from build123d import *

# Parameters (mm, degrees)
BOSS_EXTRU_1_DEPTH      = 8
ENL_V_MAT_EXTRU_1_DEPTH = 5
ESQUISSE4_W             = 5
ESQUISSE4_H             = 1
BOSS_EXTRU_3_DEPTH      = 0.48904
ESQUISSE5_W             = 1
ESQUISSE5_H             = 5
BOSS_EXTRU_4_DEPTH      = 0.48904
ESQUISSE6_W             = 1
ESQUISSE6_H             = 5
BOSS_EXTRU_5_DEPTH      = 0.48904
ESQUISSE7_W             = 1
ESQUISSE7_H             = 5
BOSS_EXTRU_6_DEPTH      = 0.48904
ESQUISSE8_W             = 5
ESQUISSE8_H             = 1
BOSS_EXTRU_7_DEPTH      = 0.48904
ESQUISSE9_W             = 5
ESQUISSE9_H             = 1
BOSS_EXTRU_8_DEPTH      = 0.48904
ESQUISSE10_W            = 3
ESQUISSE10_H            = 36.5
ENL_V_MAT_EXTRU_3_DEPTH = 99.707699801
ESQUISSE11_W            = 41.5
ESQUISSE11_H            = 3
ENL_V_MAT_EXTRU_4_DEPTH = 99.686422572
ESQUISSE12_W            = 11
ESQUISSE12_H            = 3
ENL_V_MAT_EXTRU_5_DEPTH = 99.686422572


with BuildPart() as part:
    # Esquisse1 → Boss.-Extru.1 (new body)
    with BuildSketch(Plane.XY):
        with BuildLine():
            Line((2, 0), (67, 0))
            ThreePointArc((67, 0), (68.414213562, 0.585786438), (69, 2))
            Line((69, 2), (69, 69.1))
            ThreePointArc((69, 69.1), (68.414213562, 70.514213562), (67, 71.1))
            Line((67, 71.1), (2, 71.1))
            ThreePointArc((2, 71.1), (0.585786438, 70.514213562), (0, 69.1))
            Line((0, 69.1), (0, 2))
            ThreePointArc((0, 2), (0.585786438, 0.585786438), (2, 0))
        make_face()
    extrude(amount=BOSS_EXTRU_1_DEPTH)

    # Esquisse3 → Enlèv. mat.-Extru.1 (cut)
    with BuildSketch(Plane.XY.offset(8)):
        with BuildLine():
            Line((2, 1), (67, 1))
            ThreePointArc((67, 1), (67.707106781, 1.292893219), (68, 2))
            Line((68, 2), (68, 69.1))
            ThreePointArc((68, 69.1), (67.707106781, 69.807106781), (67, 70.1))
            Line((67, 70.1), (2, 70.1))
            ThreePointArc((2, 70.1), (1.292893219, 69.807106781), (1, 69.1))
            Line((1, 69.1), (1, 2))
            ThreePointArc((1, 2), (1.292893219, 1.292893219), (2, 1))
        make_face()
    extrude(amount=-ENL_V_MAT_EXTRU_1_DEPTH, mode=Mode.SUBTRACT)

    # Esquisse4 → Boss.-Extru.3 (add)
    with BuildSketch(Plane.XZ.offset(-70.1)):
        with Locations((10.679731729, 6.5)):
            Rectangle(ESQUISSE4_W, ESQUISSE4_H)
    extrude(amount=BOSS_EXTRU_3_DEPTH)

    # Esquisse5 → Boss.-Extru.4 (add)
    with BuildSketch(Plane.ZY.offset(-68)):
        with Locations((6.5, 63.6)):
            Rectangle(ESQUISSE5_W, ESQUISSE5_H)
    extrude(amount=BOSS_EXTRU_4_DEPTH)

    # Esquisse6 → Boss.-Extru.5 (add)
    with BuildSketch(Plane(origin=(1, 0, 0), x_dir=(0, 0, -1), z_dir=(1, 0, 0))):
        with Locations((-6.5, 62.6)):
            Rectangle(ESQUISSE6_W, ESQUISSE6_H)
    extrude(amount=BOSS_EXTRU_5_DEPTH)

    # Esquisse7 → Boss.-Extru.6 (add)
    with BuildSketch(Plane(origin=(1, 0, 0), x_dir=(0, 0, -1), z_dir=(1, 0, 0))):
        with Locations((-6.5, 8.5)):
            Rectangle(ESQUISSE7_W, ESQUISSE7_H)
    extrude(amount=BOSS_EXTRU_6_DEPTH)

    # Esquisse8 → Boss.-Extru.7 (add)
    with BuildSketch(Plane(origin=(0, 1, 0), x_dir=(1, 0, 0), z_dir=(0, 1, 0))):
        with Locations((14.5, -6.5)):
            Rectangle(ESQUISSE8_W, ESQUISSE8_H)
    extrude(amount=BOSS_EXTRU_7_DEPTH)

    # Esquisse9 → Boss.-Extru.8 (add)
    with BuildSketch(Plane(origin=(0, 1, 0), x_dir=(1, 0, 0), z_dir=(0, 1, 0))):
        with Locations((47, -6.5)):
            Rectangle(ESQUISSE9_W, ESQUISSE9_H)
    extrude(amount=BOSS_EXTRU_8_DEPTH)

    # Esquisse10 → Enlèv. mat.-Extru.3 (cut, through all)
    with BuildSketch(Plane.ZY.offset(-68)):
        with Locations((6.5, 26.25)):
            Rectangle(ESQUISSE10_W, ESQUISSE10_H)
    extrude(amount=-ENL_V_MAT_EXTRU_3_DEPTH, mode=Mode.SUBTRACT)

    # Esquisse11 → Enlèv. mat.-Extru.4 (cut, through all)
    with BuildSketch(Plane.XZ.offset(-70.1)):
        with Locations((39.25, 6.5)):
            Rectangle(ESQUISSE11_W, ESQUISSE11_H)
    extrude(amount=-ENL_V_MAT_EXTRU_4_DEPTH, mode=Mode.SUBTRACT)

    # Esquisse12 → Enlèv. mat.-Extru.5 (cut, through all)
    with BuildSketch(Plane(origin=(0, 1, 0), x_dir=(1, 0, 0), z_dir=(0, 1, 0))):
        with Locations((27.5, -6.5)):
            Rectangle(ESQUISSE12_W, ESQUISSE12_H)
    extrude(amount=-ENL_V_MAT_EXTRU_5_DEPTH, mode=Mode.SUBTRACT)


solid = part.part
The model under review builds one solid part; all positions refer to its coordinate system, in mm. A direction names the side the tool comes from. Round coordinates to 2 decimals unless told otherwise and drop trailing zeros. Loops run counter-clockwise (first coordinate to the right, second up) from the corner with the lowest first, then second, coordinate; pieces in that order, holes last. Notation, with made-up numbers: (-9.5, 1.25) -> (10.5, 1.25) arc R31 ccw to (10.5, 33.25) -> close; hole circle Ø8 at (36.25, 16.25). An arc over 180 degrees is marked (long way). One line per question, with ' | ' between items. Start each with the question number.
Item 1: Add section B-B, the plane x = 61. Write out the cut boundary in (y, z).
Item 2: Machinability: for faces 4 (the face through (54.9, 0.8, 8)), 5 (the face through (34, 1, 6)), which of the approach directions +Z, -Z, +X, -X, +Y, -Y give a long, thin tool a straight path to every point of the face, cutting with its end or side? Answer none if there is none.
Item 3: Add section C-C, the plane y = 36. Write out the cut boundary in (x, z).
Item 4: Draft analysis for pull direction Y (two halves, no side actions). For faces 1 (the face through (68.4, 0.57, 3.94)), 2 (the face through (34, 36, 3)), 3 (the face through (34, 36, 0)), state which applies: +Y half, -Y half, draft (parallel to the pull), parting line (faces both ways), or undercut.
Item 5: Add section A-A, the plane z = 4. Write out the cut boundary in (x, y), then the cut area to 3 significant figures.
Item 6: For pin 1 (0.8 mm diameter, centred on x = 30, y = 70.5, fed in from +Z); pin 2 (1.5 mm diameter, centred on x = 59, y = 10.5, fed in from +Z); pin 3 (0.8 mm diameter, centred on x = 68.5, z = 6, fed in from +Y), all flat-tipped, find the tip position at first contact; note any pin that passes through.
Item 7: Wall thickness on line 1 along X through (y, z) = (27, 3.75); line 2 along Y through (x, z) = (19, 3.75); line 3 along Z through (x, y) = (18, 67): over which ranges is each line inside the solid? List them lowest first. Write a range as [from, to].
Return value:
1) outline: (0, 0) -> (71.1, 0) -> (71.1, 8) -> (70.1, 8) -> (70.1, 3) -> (1, 3) -> (1, 8) -> (0, 8) -> close
2) face 4: +Z, +X, -X, +Y, -Y | face 5: none
3) outline: (0, 0) -> (69, 0) -> (69, 5) -> (68, 5) -> (68, 3) -> (1, 3) -> (1, 8) -> (0, 8) -> close
4) face 1: -Y half | face 2: undercut | face 3: draft
5) outline: (0, 2) arc R2 ccw to (2, 0) -> (67, 0) arc R2 ccw to (69, 2) -> (69, 69.1) arc R2 ccw to (67, 71.1) -> (2, 71.1) arc R2 ccw to (0, 69.1) -> close; hole (1, 2) arc R1 ccw to (2, 1) -> (67, 1) arc R1 ccw to (68, 2) -> (68, 69.1) arc R1 ccw to (67, 70.1) -> (2, 70.1) arc R1 ccw to (1, 69.1) -> close | area: 274 mm2
6) pin 1: stops at z = 5 | pin 2: stops at z = 3 | pin 3: stops at y = 70.77
7) line 1: x = [0, 1], [68, 69] | line 2: y = [0, 1], [70.1, 71.1] | line 3: z = [0, 3]
